Input: part model. Units: mm. Frame: model coordinates. A direction names the side the tool comes from. Give positions to 0.01 mm unless a question says otherwise; leave off trailing zeros. Loops run counter-clockwise (first coordinate to the right, second up) from the corner with the lowest first, then second, coordinate; pieces in that order, holes last. Notation, with made-up numbers: M 8.5,-40 L 51.5,-40 A17 ccw 51.5,-19 Z; hole C -37,14.5 d3. An arc over 180 degrees is marked long. Use CSV: the item, a comma, the result in double quotes. Start each with the question number.
Q1. Pin query (flat end, axial travel): pin 1 (8 mm diameter, centred on y = -653.5, z = 662.5, fed in from -X); pin 2 (4 mm diameter, centred on y = -459, z = 665, fed in from +X). Return the tip coordinate at first contact, or that it passes through.
Q2. Section B-B, the plane z = 631. Output: boundary loops of the cut face in (x, y).
Q3. Material intervals for line 1 along Z through (x, y) = (127.5, -405); line 2 along Y through (x, z) = (1022.5, 827); line 3 along X through (y, z) = (-766.5, 341.5), sorted ascending.
Q4. Section A-A, the plane x = 1220. Output: boundary loops of the cut face in (y, z), plus the area to 3 significant figures.
Q5. Pull-direction query (X, two-part tool) for faces 1 (the cylindrical face through (110.55, -950.7, 399.903)), 2 (the flat face through (0, -439, 460)), 3 (the flat face through (1014, 0, 506)), 4 (the flat face through (2000, 25, 492)); classes: released by +X, released by -X, zero draft, split by the parting line, or undercut.
Q6. Reachability of faces 5 (the flat face through (264.456, -493, 500)), 6 (the flat face through (130, -493, 664.525)), 7 (the flat face through (134, -493, 330.571)), 8 (the flat face through (131, -900, 499)) from +Z, -Z, +X, -X, +Y, -Y: full face, straight path, thin tool, end or side. Return the list, or none.
Q7. Section C-C, the plane y = -722.5. Output: boundary loops of the cut face in (x, z).
Autodesk Inventor part; units mm, degrees
ref_plane "YZ Plane" through (0, 0, 0) normal (1, 0, 0) x (0, 1, 0)
ref_plane "XZ Plane" through (0, 0, 0) normal (0, 1, 0) x (-1, 0, 0)
ref_plane "XY Plane" through (0, 0, 0) normal (0, 0, 1) x (1, 0, 0)
sketch "Sketch1" plane through (0, 0, 0) normal (0, 1, 0) x (-1, 0, 0)
  line L0 (1000, 0) -> (1000, -0.5649)
  line L1 (1000, -0.5649) -> (0, -0.5649)
  line L2 (0, -0.5649) -> (0, 0)
  line L3 (0, -0.5649) -> (-2000, -0.5649)
  line L4 (-2000, -0.5649) -> (-2000, 999.4351)
  line L5 (-2000, 999.4351) -> (0, 999.4351)
  line L6 (0, 999.4351) -> (0, -0.5649)
  dimension "d1" = 2000
  dimension "d2" = 1000
extrude "Extrusion1" add sketch "Sketch1" along normal blind 50
sketch "Sketch2" plane through (0, 0, 0) normal (0, -1, 0) x (1, 0, 0)
  point P0 (0, 0)
sketch "Sketch3" plane through (0, 0, 0) normal (0, -1, 0) x (1, 0, 0)
  line L0 (98.4679, 994.5253) -> (98.4679, 664.5253)
  line L1 (98.4679, 330.5706) -> (98.4679, 0)
  line L2 (0, -0.5649) -> (0, 999.4351)
  line L3 (0, 664.5253) -> (264.4565, 664.5253)
  line L4 (264.4565, 664.5253) -> (264.4565, 330.5706)
  line L5 (264.4565, 330.5706) -> (0, 330.5706)
  line L6 (0, 330.5706) -> (0, 664.5253)
  point P0 (0, 0)
  dimension "d5" = 330
extrude "Extrusion2" add sketch "Sketch3" along normal blind 1000
sketch "Sketch4" plane through (0, -1000, 0) normal (0, -1, 0) x (1, 0, 0)
  line L0 (0, 664.5253) -> (264.4565, 664.5253)
  line L1 (132.2283, 664.5253) -> (132.2283, 497.5253)
  circle A0 centre (132.2283, 497.5253) radius 100
  point P0 (0, 0)
  dimension "d8" = 167
  dimension "d9" = 200
extrude "Extrusion3" cut sketch "Sketch4" against normal blind 100
sketch "Sketch5" plane through (0, 0, 0) normal (0, -1, 0) x (1, 0, 0)
  point P0 (0, 0)
equation "\"BendRadius\" = Thickness"
equation "\"BendReliefWidth\" = Thickness"
equation "\"BendReliefDepth\" = 0.5 * Thickness"
equation "\"CornerReliefSize\" = 4 * Thickness"
equation "\"MinimumRemnant\" = 2 * Thickness"
equation "\"TransitionRadius\" = BendRadius"
equation "\"JacobiRadiusSize\" = BendRadius"
equation "\"GapSize\" = Thickness"
A:
1,pin 1,"x = 0"
1,pin 2,"x = 264.46"
2,outline,"M 0,-1000 L 264.46,-1000 L 264.46,0 L 2000,0 L 2000,50 L 0,50 Z"
3,line 1,"330.57 to 664.53"
3,line 2,"0 to 50"
3,line 3,"0 to 264.46"
4,outline,"M 0,-0.56 L 50,-0.56 L 50,999.44 L 0,999.44 Z"
4,area,"50,000 mm^2"
5,face 1,"undercut"
5,face 2,"released by -X"
5,face 3,"zero draft"
5,face 4,"released by +X"
6,face 5,"+Z, -Z, +X, -Y"
6,face 6,"+Z, +X, -X, -Y"
6,face 7,"-Z, +X, -X, -Y"
6,face 8,"-Y"
7,outline,"M 0,330.57 L 264.46,330.57 L 264.46,664.53 L 0,664.53 Z"
